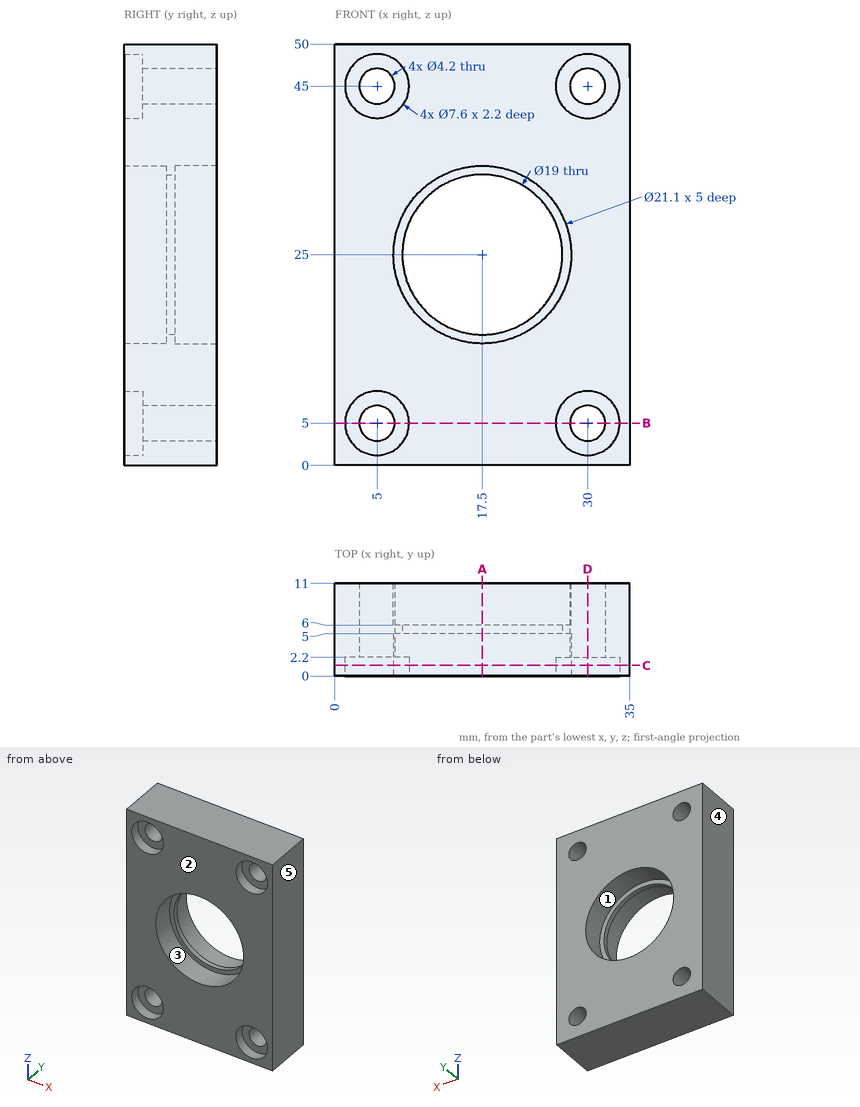
Job drawing, mm, ordinate dimensions from the low corner. One solid piece. A direction names the side the tool comes from. Give positions to 0.01 mm unless a question says otherwise; leave off trailing zeros. Loops run counter-clockwise (first coordinate to the right, second up) from the corner with the lowest first, then second, coordinate; pieces in that order, holes last. Notation, with made-up numbers: M 10,-34.5 L 32,-34.5 A12 cw 32,-19.5 Z; hole C 80,84.25 d11. An arc over 180 degrees is marked long. Return JSON: item names as keys, results as strings.
1) Flat gauge pin, fed straight in: pin 1 Ø4.5 at (x, z) = (5, 45) entering from -Y. Where does the tip first touch, or does it go through?
Calculated:
{"pin 1": "stops at y = 2.2"}
2) Pull direction X, two halves, no side cores. Call the marked faces 3, 4 and 5: released by +X, released by -X, zero draft, split by the parting line, or undercut.
Calculated:
{"face 3": "undercut", "face 4": "released by -X", "face 5": "released by +X"}
3) Saw through at B-B, the plane z = 5. List the corners of the cut face in (x, y).
Calculated:
{"outline": "M 0,0 L 1.2,0 L 1.2,2.2 L 2.9,2.2 L 2.9,11 L 0,11 Z; M 7.1,2.2 L 8.8,2.2 L 8.8,0 L 26.2,0 L 26.2,2.2 L 27.9,2.2 L 27.9,11 L 7.1,11 Z; M 32.1,2.2 L 33.8,2.2 L 33.8,0 L 35,0 L 35,11 L 32.1,11 Z"}
4) Saw through at D-D, the plane x = 30. List the corners of the cut face in (y, z), then the cut area to 3 significant figures.
Calculated:
{"outline": "M 0,0 L 11,0 L 11,2.9 L 2.2,2.9 L 2.2,1.2 L 0,1.2 Z; M 0,8.8 L 2.2,8.8 L 2.2,7.1 L 11,7.1 L 11,42.9 L 2.2,42.9 L 2.2,41.2 L 0,41.2 Z; M 0,48.8 L 2.2,48.8 L 2.2,47.1 L 11,47.1 L 11,50 L 0,50 Z", "area": "443 mm2"}
5) 3-axis set-ups, long thin cutter, end or side, ignore diameter. For the marked faces 1 and 2: which of +Z, -Z, +X, -X, +Y, -Y reach the whole face in a straight line?
Calculated:
{"face 1": "+Y", "face 2": "+Z, -Z, +X, -X, -Y"}
6) Saw through at C-C, the plane y = 1.25. List the corners of the cut face in (x, z), then the cut area to 3 significant figures.
Calculated:
{"outline": "M 0,0 L 35,0 L 35,50 L 0,50 Z; hole C 5,5 d7.6; hole C 5,45 d7.6; hole C 17.5,25 d21.1; hole C 30,5 d7.6; hole C 30,45 d7.6", "area": "1,220 mm2"}
7) Drill centre lines: line 1 (X direction, y = 7, z = 45); line 2 (X direction, y = 1.55, z = 5); line 3 (Z direction, x = 29, y = 2). Where is each one in solid material? Low to high.
Calculated:
{"line 1": "x = 0 to 2.9, 7.1 to 27.9, 32.1 to 35", "line 2": "x = 0 to 1.2, 8.8 to 26.2, 33.8 to 35", "line 3": "z = 0 to 1.33, 8.67 to 41.33, 48.67 to 50"}
8) Saw through at A-A, the plane x = 17.5. List the corners of the cut face in (y, z).
Calculated:
{"outline": "M 0,0 L 11,0 L 11,14.45 L 6,14.45 L 6,15.5 L 5,15.5 L 5,14.45 L 0,14.45 Z; M 0,35.55 L 5,35.55 L 5,34.5 L 6,34.5 L 6,35.55 L 11,35.55 L 11,50 L 0,50 Z"}
